Could you check a few things on this drawing? It's one solid part, dimensions in mm from its lowest x, y, z. Give positions to 0.01 mm unless a question says otherwise; leave off trailing zeros. Loops run counter-clockwise (first coordinate to the right, second up) from the corner with the lowest first, then second, coordinate; pieces in that order, holes last. Notation, with made-up numbers: M -15.5,16 L 15.5,16 A17 ccw 15.5,25 Z; hole C 73.25,68 d10. An arc over 180 degrees is marked long. Return JSON: item names as keys, results as strings. Group by question number.
1. Please list where these lines run through material, in increasing order: line 1 (X direction, y = 1.4, z = 10); line 2 (Z direction, x = 40, y = 0.7); line 3 (X direction, y = 0.8, z = 36).
2. If we section it at D-D (x = 40): Write out the boundary of the cut face in (y, z), plus the area to 3 significant figures.
3. If we section it at A-A (x = 22): Write out the boundary of the cut face in (y, z).
4. If we section it at C-C (z = 36): Write out the boundary of the cut face in (x, y).
5. For pin 1 (6.5 mm diameter, centred on x = 22, z = 10, fed in from -Y), with a flat end and sliding along its axis, tell me the tip position at first contact or that it passes through.
6. If we section it at B-B (y = 0.65): Write out the boundary of the cut face in (x, z).
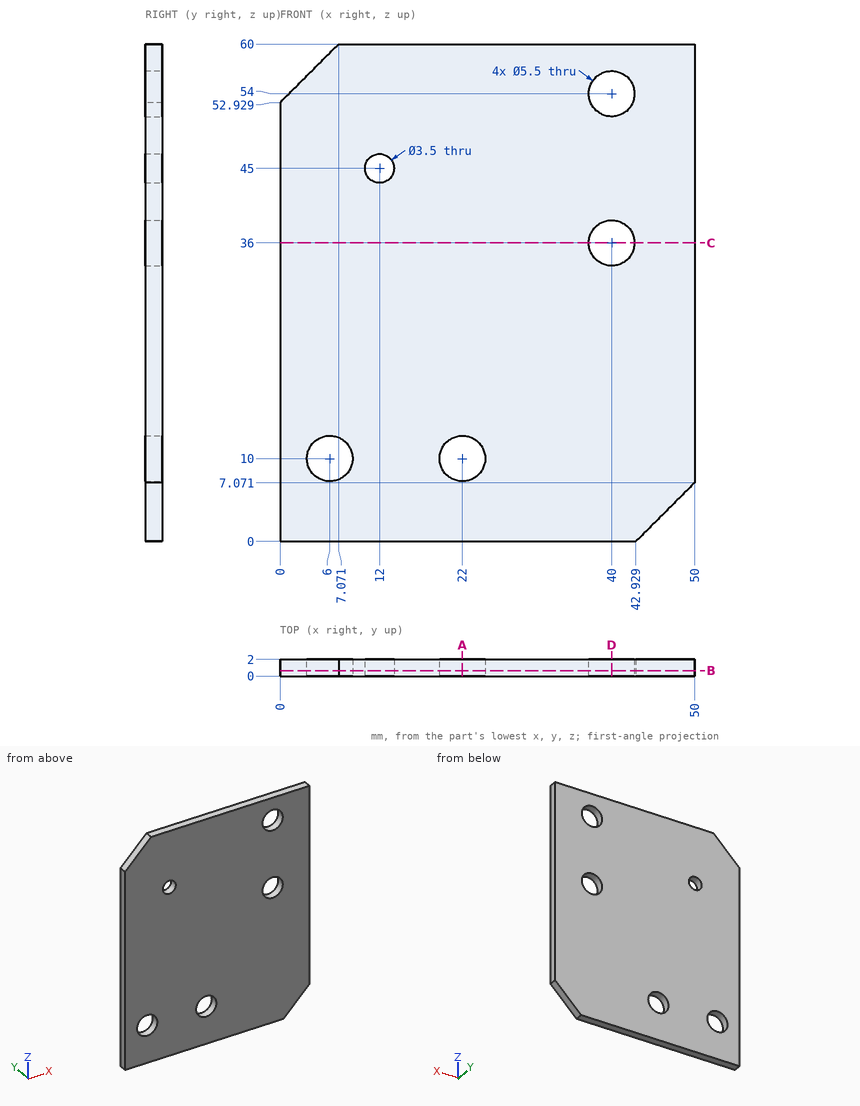
Answer:
{
 "1": {"line 1": "x = 0 to 3.25, 8.75 to 19.25, 24.75 to 50", "line 2": "z = 0 to 33.25, 38.75 to 51.25, 56.75 to 60", "line 3": "x = 0 to 37.25, 42.75 to 50"},
 "2": {"outline": "M 0,0 L 2,0 L 2,33.25 L 0,33.25 Z; M 0,38.75 L 2,38.75 L 2,51.25 L 0,51.25 Z; M 0,56.75 L 2,56.75 L 2,60 L 0,60 Z", "area": "98.0 mm²"},
 "3": {"outline": "M 0,0 L 2,0 L 2,7.25 L 0,7.25 Z; M 0,12.75 L 2,12.75 L 2,60 L 0,60 Z"},
 "4": {"outline": "M 0,0 L 37.25,0 L 37.25,2 L 0,2 Z; M 42.75,0 L 50,0 L 50,2 L 42.75,2 Z"},
 "5": {"pin 1": "stops at y = 0"},
 "6": {"outline": "M 0,0 L 42.93,0 L 50,7.07 L 50,60 L 7.07,60 L 0,52.93 Z; hole C 6,10 d5.5; hole C 12,45 d3.5; hole C 22,10 d5.5; hole C 40,36 d5.5; hole C 40,54 d5.5"}
}
